The listing builds one solid part. Answer for the finished solid, in the listing's coordinates (mm). A direction names the side the tool comes from. Coordinates: 2 decimals unless noted, no trailing zeros. Order: outer loops, then holes, each group sorted by start corner. A loop starts at its lowest first (then second) coordinate and runs counter-clockwise, first axis right, second up.
from build123d import *

# Parameters (mm, degrees)
SKETCH_2_W          = 102.444219067
SKETCH_2_H          = 95.84178499
CUT_EXTRUDE_1_DEPTH = 4


with BuildPart() as part:
    # Sketch 1 → Revolve 1 (revolve)
    with BuildSketch(Plane.XY, mode=Mode.PRIVATE) as revolve_1_sk:
        Polygon((8, 21.3), (8, 10), (12.5, 10), (12.5, 0), (15.835, 0), (18, 2.165), (18, 12.3), (26.5, 12.3), (26.5, 16.3), (23.752522581, 17.3), (16.765, 17.3), (16.765, 19.535), (15, 21.3), align=None)
    revolve(revolve_1_sk.sketch.rotate(Axis((0, 0, 0), (0, 1, 0)), 270), axis=Axis((0, 0, 0), (0, 1, 0)))

    # Sketch 2 → Cut-Extrude 1 (cut)
    with BuildSketch(Plane(origin=(0, 21.3, 0), x_dir=(1, 0, 0), z_dir=(0, 1, 0))):
        with Locations((3.088235295, -0.106490872)):
            Rectangle(SKETCH_2_W, SKETCH_2_H)
        Polygon((-15, 8.660254038), (-15, -8.660254038), (0, -17.320508076), (15, -8.660254038), (15, 8.660254038), (0, 17.320508076), align=None, mode=Mode.SUBTRACT)
    extrude(amount=-CUT_EXTRUDE_1_DEPTH, mode=Mode.SUBTRACT)


solid = part.part
(1) A tool of negligible diameter and unlimited length cuts with its end or side. For faces 1 (the flat face through (16, 17.3, 0)), 2 (the cylindrical face through (0.014, 18.433, -16.765)), 3 (the flat face through (15, 19, 0)), 4 (the cylindrical face through (-14.526, 18.433, 8.37)), 5 (the cylindrical face through (14.512, 18.433, 8.395)), from which of +Z, -Z, +X, -X, +Y, -Y can it reach the whole face along a straight path? Write none if from no direction.
(2) The mould has two halves that part along X. Classify faces 6 (the cylindrical face through (-7.81, 15.57, -1.73)), 7 (the flat face through (-15, 19, 0)), 8 (the cylindrical face through (-0.014, 18.433, 16.765)): pulls with the +X half, pulls with the -X half, needs draft (parallel to the pull), parting line crosses it, or undercut.
(3) Find section C-C on y = 8.5. Determine the outline of the cut face in (x, z).
(4) Given pin 1 Ø1.2 at (y, z) = (19.5, 1) entering from -X; pin 2 Ø3 at (y, z) = (12.5, 3.5) entering from -X; pin 3 Ø1.5 at (x, z) = (-6, 1.5) entering from -Y; pin 4 Ø6 at (y, z) = (7, 18) entering from +X, each flat-ended and moving along its own axis, determine where each tip first touches the part or whether it passes through.
(5) Find the intervals of material crossed by probe 1 along X at (y, z) = (16, 0); probe 2 along Y at (x, z) = (-15.5, 20); probe 3 along Z at (x, y) = (-4, 2), in increasing order.
(6) Find section A-A on x = 0. Determine the outline of the cut face in (y, z) (3 decimals), then the cut area to 3 significant figures.
(7) Find section B-B on y = 13.75. Determine the outline of the cut face in (x, z).
Resolved:
1. face 1: +Y
1. face 2: -Z, +Y
1. face 3: +Z, -Z, +X, +Y
1. face 4: +Z, -X, +Y
1. face 5: +Z, +X, +Y
2. face 6: undercut
2. face 7: pulls with the -X half
2. face 8: parting line crosses it
3. outline: circle Ø36 at (0, 0); hole circle Ø25 at (0, 0)
4. pin 1: stops at x = -15
4. pin 2: stops at x = -26.42
4. pin 3: passes through
4. pin 4: stops at x = 9.95
5. probe 1: x = -26.5 to -8, 8 to 26.5
5. probe 2: y = 12.3 to 16.74
5. probe 3: z = -17.38 to -11.84, 11.84 to 17.38
6. outline: (0, -15.835) - (2.165, -18) - (12.3, -18) - (12.3, -26.5) - (16.3, -26.5) - (17.3, -23.753) - (17.3, -16.765) - (19.535, -16.765) - (21.3, -15) - (21.3, -8) - (10, -8) - (10, -12.5) - (0, -12.5) - close; (0, 12.5) - (10, 12.5) - (10, 8) - (21.3, 8) - (21.3, 15) - (19.535, 16.765) - (17.3, 16.765) - (17.3, 23.753) - (16.3, 26.5) - (12.3, 26.5) - (12.3, 18) - (2.165, 18) - (0, 15.835) - close
6. area: 401 mm2
7. outline: circle Ø53 at (0, 0); hole circle Ø16 at (0, 0)
